Drawing for the job (mm, zero at the part's lowest x, y, z). Coordinates: 2 decimals unless noted, no trailing zeros. Order: outer loops, then holes, each group sorted by start corner. A loop starts at its lowest first (then second) coordinate and runs counter-clockwise, first axis right, second up. Notation, with made-up numbers: (60, 82) -> (103, 82) arc R23 ccw to (103, 118) -> close; hole circle Ø3 at (59.25, -9.75). An arc over 180 degrees is marked (long way). Write each question's results on one line, items separated by ' | '.
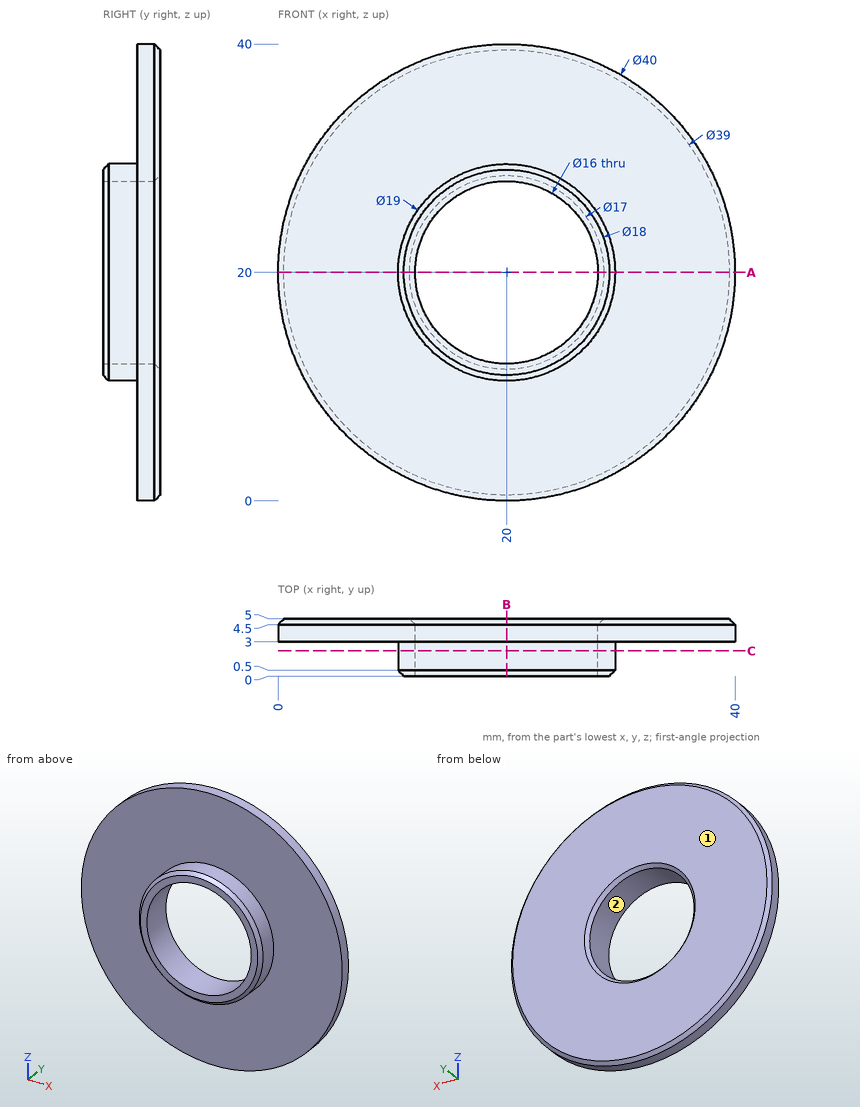
Item 1: Pull direction Z, two halves, no side cores. Call the marked faces 1 and 2: released by +Z, released by -Z, zero draft, split by the parting line, or undercut.
Answer:
face 1: zero draft | face 2: undercut
Item 2: Slice it at C-C, the plane y = 2.2. List the corners of the cut face in (x, z).
Answer:
outline: circle Ø19 at (20, 20); hole circle Ø16 at (20, 20)
Item 3: Pin check, flat tips, straight feed: pin 1 (3 mm diameter, centred on x = 19, y = 1, fed in from +Z); pin 2 (1 mm diameter, centred on x = 8.5, z = 11.5, fed in from -Y); pin 3 (2 mm diameter, centred on x = 31.5, y = 0.5, fed in from -Z); pin 4 (1 mm diameter, centred on x = 16, y = 1, fed in from +Z). Stop position of each tip, or through.
Answer:
pin 1: stops at z = 29.5 | pin 2: stops at y = 3 | pin 3: passes through | pin 4: stops at z = 28.83
Item 4: Drill centre lines: line 1 (Z direction, x = 20, y = 1.9); line 2 (X direction, y = 3.1, z = 20). Where is each one in solid material? Low to high. Write a range as from..to.
Answer:
line 1: z = 10.5..12, 28..29.5 | line 2: x = 0..12, 28..40
Item 5: Slice it at B-B, the plane x = 20. List the corners of the cut face in (y, z).
Answer:
outline: (0, 11) -> (0.5, 10.5) -> (3, 10.5) -> (3, 0) -> (4.5, 0) -> (5, 0.5) -> (5, 11.5) -> (4.5, 12) -> (0, 12) -> close; (0, 28) -> (4.5, 28) -> (5, 28.5) -> (5, 39.5) -> (4.5, 40) -> (3, 40) -> (3, 29.5) -> (0.5, 29.5) -> (0, 29) -> close
Item 6: Slice it at A-A, the plane z = 20. List the corners of the cut face in (x, y).
Answer:
outline: (0, 3) -> (10.5, 3) -> (10.5, 0.5) -> (11, 0) -> (12, 0) -> (12, 4.5) -> (11.5, 5) -> (0.5, 5) -> (0, 4.5) -> close; (28, 0) -> (29, 0) -> (29.5, 0.5) -> (29.5, 3) -> (40, 3) -> (40, 4.5) -> (39.5, 5) -> (28.5, 5) -> (28, 4.5) -> close
